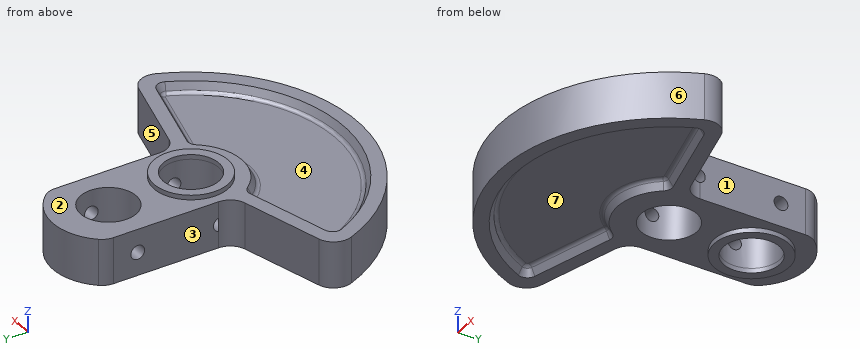
```python
from build123d import *

# Parameters (mm, degrees)
SKETCH1_R            = 6
BOSS_EXTRUDE1_DEPTH  = 5
CUT_EXTRUDE1_DEPTH   = 2
CUT_EXTRUDE1_DRAFT   = -30
FILLET1_R            = 1
MIRROR2_COPY_1_DEPTH = 2
MIRROR2_COPY_1_DRAFT = -30
FILLET1_OF_MIRROR2_R = 1
SKETCH3_R            = 8
SKETCH3_R_2          = 6
BOSS_EXTRUDE2_DEPTH  = 1
SKETCH4_R            = 8
SKETCH4_R_2          = 6
BOSS_EXTRUDE3_DEPTH  = 1
SKETCH5_R            = 1.5
CUT_EXTRUDE2_DEPTH   = 57.883602865


with BuildPart() as part:
    # Sketch1 → Boss-Extrude1 (new, symmetric)
    with BuildSketch(Plane.XY):
        with BuildLine():
            Line((-10, 23.291502622), (-10, 0.389816028))
            ThreePointArc((-10, 0.389816028), (-10.826586639, -2.045229688), (-12.96472382, -3.473887278))
            Line((-12.96472382, -3.473887278), (-30.667194256, -8.217249935))
            ThreePointArc((-30.667194256, -8.217249935), (-33.214466382, -10.301810854), (-33.335907835, -13.591072395))
            ThreePointArc((-33.335907835, -13.591072395), (0, -36), (33.335907835, -13.591072395))
            ThreePointArc((33.335907835, -13.591072395), (33.214466382, -10.301810854), (30.667194256, -8.217249935))
            Line((30.667194256, -8.217249935), (12.96472382, -3.473887278))
            ThreePointArc((12.96472382, -3.473887278), (10.826586639, -2.045229688), (10, 0.389816028))
            Line((10, 0.389816028), (10, 23.291502622))
            ThreePointArc((10, 23.291502622), (9.741657387, 24.705716185), (9, 25.937253933))
            ThreePointArc((9, 25.937253933), (0, 30), (-9, 25.937253933))
            ThreePointArc((-9, 25.937253933), (-9.741657387, 24.705716185), (-10, 23.291502622))
        make_face()
        Circle(SKETCH1_R, mode=Mode.SUBTRACT)
        with Locations((0, 18)):
            Circle(SKETCH1_R, mode=Mode.SUBTRACT)
    extrude(amount=BOSS_EXTRUDE1_DEPTH, both=True)


with BuildPart() as cut_extrude1_tool:
    # Sketch2 → Cut-Extrude1 (with draft: the straight prism first)
    with BuildSketch(Plane.XY.offset(5)):
        with BuildLine():
            ThreePointArc((-28.775190686, -10.816117648), (-30.064835096, -11.891388911), (-30.080620505, -13.570418933))
            ThreePointArc((-30.080620505, -13.570418933), (0, -33), (30.080620505, -13.570418933))
            ThreePointArc((30.080620505, -13.570418933), (30.064835096, -11.891388911), (28.775190686, -10.816117648))
            Line((28.775190686, -10.816117648), (10.81465278, -6.00360602))
            ThreePointArc((10.81465278, -6.00360602), (9.656117125, -6.040925986), (8.712858584, -6.714618031))
            ThreePointArc((8.712858584, -6.714618031), (0, -11), (-8.712858584, -6.714618031))
            ThreePointArc((-8.712858584, -6.714618031), (-9.656117125, -6.040925986), (-10.81465278, -6.00360602))
            Line((-10.81465278, -6.00360602), (-28.775190686, -10.816117648))
        make_face()
    extrude(amount=-CUT_EXTRUDE1_DEPTH)
    # Cut-Extrude1: the draft: its side faces are tilted about the plane it starts from
    cut_extrude1_sides = [cut_extrude1_tool.faces().sort_by_distance(p)[0] for p in [
        (-9.656117125, -6.040925986, 4),
        (-19.794921733, -8.409861834, 4),
        (-30.064835096, -11.891388911, 4),
        (0, -33, 4),
        (30.064835096, -11.891388911, 4),
        (19.794921733, -8.409861834, 4),
        (9.656117125, -6.040925986, 4),
        (0, -11, 4),
    ]]
    draft(cut_extrude1_sides, Plane.XY.offset(5), CUT_EXTRUDE1_DRAFT)


with BuildPart() as part_1:
    add(part.part)

    # Cut-Extrude1: cut by cut_extrude1_tool
    add(cut_extrude1_tool.part, mode=Mode.SUBTRACT)

    # Fillet1
    fillet1_edges = [part_1.edges().sort_by_distance(p)[0] for p in [
        (29.021400058, -12.385935829, 3),
        (0, -31.845299462, 3),
        (-29.021400058, -12.385935829, 3),
        (-19.496063242, -9.525216906, 3),
        (-10.026139506, -7.134734365, 3),
        (0, -12.154700538, 3),
        (10.026139506, -7.134734365, 3),
        (19.496063242, -9.525216906, 3),
    ]]
    fillet(fillet1_edges, radius=FILLET1_R)


with BuildPart() as mirror2_copy_1_tool:
    # Mirror2 copy 1 sketch → Mirror2 copy 1 (with draft: the straight prism first)
    with BuildSketch(Plane(origin=(0, 0, -5), x_dir=(1, 0, 0), z_dir=(0, 0, -1))):
        with BuildLine():
            ThreePointArc((-28.775190686, 10.816117648), (-30.064835096, 11.891388911), (-30.080620505, 13.570418933))
            ThreePointArc((-30.080620505, 13.570418933), (0, 33), (30.080620505, 13.570418933))
            ThreePointArc((30.080620505, 13.570418933), (30.064835096, 11.891388911), (28.775190686, 10.816117648))
            Line((28.775190686, 10.816117648), (10.81465278, 6.00360602))
            ThreePointArc((10.81465278, 6.00360602), (9.656117125, 6.040925986), (8.712858584, 6.714618031))
            ThreePointArc((8.712858584, 6.714618031), (0, 11), (-8.712858584, 6.714618031))
            ThreePointArc((-8.712858584, 6.714618031), (-9.656117125, 6.040925986), (-10.81465278, 6.00360602))
            Line((-10.81465278, 6.00360602), (-28.775190686, 10.816117648))
        make_face()
    extrude(amount=-MIRROR2_COPY_1_DEPTH)
    # Mirror2 copy 1: the draft: its side faces are tilted about the plane it starts from
    mirror2_copy_1_sides = [mirror2_copy_1_tool.faces().sort_by_distance(p)[0] for p in [
        (-9.656117125, -6.040925986, -4),
        (-19.794921733, -8.409861834, -4),
        (-30.064835096, -11.891388911, -4),
        (0, -33, -4),
        (30.064835096, -11.891388911, -4),
        (19.794921733, -8.409861834, -4),
        (9.656117125, -6.040925986, -4),
        (0, -11, -4),
    ]]
    draft(mirror2_copy_1_sides, Plane(origin=(0, 0, -5), x_dir=(1, 0, 0), z_dir=(0, 0, -1)), MIRROR2_COPY_1_DRAFT)


with BuildPart() as part_2:
    add(part_1.part)

    # Mirror2 copy 1: cut by mirror2_copy_1_tool
    add(mirror2_copy_1_tool.part, mode=Mode.SUBTRACT)

    # Fillet1 of Mirror2
    fillet1_of_mirror2_edges = [part_2.edges().sort_by_distance(p)[0] for p in [
        (29.021400058, -12.385935829, -3),
        (0, -31.845299462, -3),
        (-29.021400058, -12.385935829, -3),
        (-19.496063242, -9.525216906, -3),
        (-10.026139506, -7.134734365, -3),
        (0, -12.154700538, -3),
        (10.026139506, -7.134734365, -3),
        (19.496063242, -9.525216906, -3),
    ]]
    fillet(fillet1_of_mirror2_edges, radius=FILLET1_OF_MIRROR2_R)

    # Sketch3 → Boss-Extrude2 (add)
    with BuildSketch(Plane(origin=(0, 0, -5), x_dir=(-1, 0, 0), z_dir=(0, 0, -1))):
        with Locations((0, 18)):
            Circle(SKETCH3_R)
        with Locations((0, 18)):
            Circle(SKETCH3_R_2, mode=Mode.SUBTRACT)
    extrude(amount=BOSS_EXTRUDE2_DEPTH)

    # Sketch4 → Boss-Extrude3 (add)
    with BuildSketch(Plane.XY.offset(5)):
        with Locations(Location((0, 0, 0), (0, 0, 180))):
            Circle(SKETCH4_R)
        Circle(SKETCH4_R_2, mode=Mode.SUBTRACT)
    extrude(amount=BOSS_EXTRUDE3_DEPTH)

    # Sketch5 → Cut-Extrude2 (cut, through all)
    with BuildSketch(Plane.ZY.offset(10)):
        with Locations((0, 18)):
            Circle(SKETCH5_R)
        Circle(SKETCH5_R)
    extrude(amount=-CUT_EXTRUDE2_DEPTH, mode=Mode.SUBTRACT)


solid = part_2.part
```
CAD build for the part. Positions are in the model's coordinates, mm. Face numbers are marked on the shaded views. A direction names the side the tool comes from. Round coordinates to 2 decimals unless told otherwise and drop trailing zeros. Write each loop counter-clockwise with the first axis right and the second up, starting at its lowest first coordinate (ties: lowest second). Pieces come first, ordered by that corner, then holes. Notation, with made-up numbers: M -39,43.25 L -10,43.25 A22 cw -10,80.25 Z; hole C -34,64.5 d8. An arc over 180 degrees is marked long. One line per question, with ' | ' between items.
1. Cut at D-D on y = 3.5. Write the cut outline in (x, z).
Working result:
outline: M -10,-5 L -4.87,-5 L -4.87,6 L -7.19,6 L -7.19,5 L -10,5 Z; M 4.87,-5 L 10,-5 L 10,5 L 7.19,5 L 7.19,6 L 4.87,6 Z
2. Probe L1, parallel to Y at x = 7.25, z = 0; L2, parallel to Y at x = 0, z = -5.8; L3, parallel to X at y = 18, z = 2.75. List the from-to ranges inside material, lowest first. Write a range as from..to.
Working result:
L1: -35.26..-1.5, 1.5..16.5, 19.5..27.56 | L2: 10..12, 24..26 | L3: -10..-6, 6..10
3. Which spindle directions (+Z, -Z, +X, -X, +Y, -Y) get a long thin tool onto all of the face, cutting with end or side? Do the marked faces 1, 2 and 3. Say none if no direction does.
Working result:
face 1: +Z, -Z, +X, +Y | face 2: +Z | face 3: +Z, -Z, -X, +Y
4. Cut at C-C on x = 0. Count the separate pieces of the cut face and the enclosed holes in it, and give its area (3 significant figures).
Working result:
separate pieces: 3 | enclosed holes: 0 | area: 345 mm2
5. Cut at B-B on y = 18. Write the cut outline in (x, z).
Working result:
outline: M -10,-5 L -8,-5 L -8,-6 L -6,-6 L -6,-1.5 L -10,-1.5 Z; M -10,1.5 L -6,1.5 L -6,5 L -10,5 Z; M 6,-6 L 8,-6 L 8,-5 L 10,-5 L 10,-1.5 L 6,-1.5 Z; M 6,1.5 L 10,1.5 L 10,5 L 6,5 Z
6. Pin check, flat tips, straight feed: pin 1 Ø3.5 at (y, z) = (0, 0) entering from +X; pin 2 Ø8 at (x, y) = (-17.5, -23) entering from -Z; pin 3 Ø14 at (x, y) = (0, 0) entering from -Z. Stop position of each tip, or through.
Working result:
pin 1: x = 10.62 | pin 2: z = -4.83 | pin 3: z = -5
7. Mould opens along X. For the marked faces 4, 5, 6 and 7 say: pulls with the +X half, pulls with the -X half, needs draft (parallel to the pull), parting line crosses it, or undercut.
Working result:
face 4: undercut | face 5: pulls with the +X half | face 6: parting line crosses it | face 7: undercut
8. Cut at A-A on z = 0. Write the cut outline in (x, y), and give its area (3 significant figures).
Working result:
outline: M -33.34,-13.59 A36 ccw 33.34,-13.59 A4 ccw 30.67,-8.22 L 12.96,-3.47 A4 cw 10.47,-1.5 L 5.81,-1.5 A6 cw -5.81,-1.5 L -10,-1.5 L -10,0.39 A4 cw -12.96,-3.47 L -30.67,-8.22 A4 ccw Z; M -10,1.5 L -5.81,1.5 A6 cw 5.81,1.5 L 10,1.5 L 10,16.5 L 5.81,16.5 A6 cw -5.81,16.5 L -10,16.5 Z; M -10,19.5 L -5.81,19.5 A6 cw 5.81,19.5 L 10,19.5 L 10,23.29 A4 ccw 9,25.94 A12 ccw -9,25.94 A4 ccw -10,23.29 Z | area: 2,010 mm2
